from build123d import *

# Parameters (mm, degrees)
SKETCH1_W      = 5
SKETCH1_H      = 4
SKETCH2_R      = 3
EXTRUDE1_DEPTH = 12
EXTRUDE2_DEPTH = 3
CHAMFER1_SIZE  = 0.6135
FILLET1_R      = 0.2


with BuildPart() as part:
    # Sketch1 → Revolve1 (revolve)
    with BuildSketch(Plane.XZ.offset(-21.5)):
        with Locations((-13, -2.4)):
            Rectangle(SKETCH1_W, SKETCH1_H)
    revolve(axis=Axis((-15.5, 21.5, -0.4), (0, 0, -1)))

    # Sketch2 → Extrude1 (add)
    with BuildSketch(Plane(origin=(0, 0, -4.4), x_dir=(-1, 0, 0), z_dir=(0, 0, -1))):
        with Locations((15.5, 21.5)):
            Circle(SKETCH2_R)
    extrude(amount=EXTRUDE1_DEPTH)

    # Sketch3 → Extrude2 (cut)
    with BuildSketch(Plane.XY.offset(-0.4)):
        Polygon((-17.5, 22.654700538), (-17.5, 20.345299462), (-15.5, 19.190598923), (-13.5, 20.345299462), (-13.5, 22.654700538), (-15.5, 23.809401077), align=None)
    extrude(amount=-EXTRUDE2_DEPTH, mode=Mode.SUBTRACT)

    # Sketch4 → Cut-Revolve1 (revolve, cut)
    with BuildSketch(Plane.XZ.offset(-21.5)):
        Polygon((-13.5, -3.4), (-15.5, -3.4), (-15.5, -4.127940469), align=None)
    revolve(axis=Axis((-15.5, 21.5, -3.399975), (0, 0, -1)), mode=Mode.SUBTRACT)

    # Chamfer1
    chamfer1_edges = [part.edges().sort_by_distance(p)[0] for p in [
        (-12.5, 21.5, -16.4),
    ]]
    chamfer(chamfer1_edges, length=CHAMFER1_SIZE)

    # Fillet1
    fillet1_edges = [part.edges().sort_by_distance(p)[0] for p in [
        (-12.5, 21.5, -4.4),
    ]]
    fillet(fillet1_edges, radius=FILLET1_R)


solid = part.part
Geometry check sheet. Reference: the model listing, model coordinates, mm. A direction names the side the tool comes from. Round coordinates to 2 decimals unless told otherwise and drop trailing zeros. Order: outer loops, then holes, each group sorted by start corner. A loop starts at its lowest first (then second) coordinate and runs counter-clockwise, first axis right, second up. Notation, with made-up numbers: M 39,75.25 L 51,75.25 A21 ccw 51,107.25 Z; hole C 10.5,89 d3. An arc over 180 degrees is marked long. Write each question's results on one line, items separated by ' | '. Start each with the question number.
1. Cross-section at B-B on y = 18. Record the boundary of the cut face in (x, z).
2. Go/stop test with flat-tipped pins: P1, Ø0.7, axis at y = 22, z = -2.5, coming from the +X side; P2, Ø4, axis at y = 24, z = -6.5, coming from the +X side; P3, Ø6, axis at y = 19.5, z = -9.5, coming from the -X side. Record where each tip stops, or that it passes through.
3. Set-up check for faces 1 (the face through (-18, 21, -0.4)), 2 (the face through (-15, 25, -4.4)), 3 (the face through (-14.51, 19.76, -1.88)): record each of +Z, -Z, +X, -X, +Y, -Y from which the full face is reachable in a straight line by a thin tool's end or side.
4. Material ranges on L1, parallel to Z at x = -14.25, y = 17.5; L2, parallel to Y at x = -13.75, z = -2; L3, parallel to X at y = 17.5, z = -1.75, recorded low to high. Write a range as from..to.
5. Cross-section at A-A on z = -13.5. Record the boundary of the cut face in (x, y).
6. Draft check along X on faces 4 (the face through (-16.58, 26.38, -2.37)), 5 (the face through (-15.527, 21.622, -4.082)), 6 (the face through (-15, 22, -16.4)). Enter one of: pulls with the +X half, pulls with the -X half, needs draft (parallel to the pull), parting line crosses it, or undercut.
Resolved:
1) outline: M -19.07,-4.4 L -11.93,-4.4 L -11.93,-0.4 L -19.07,-0.4 Z
2) P1: x = -10.5 | P2: x = -12.54 | P3: x = -18.5
3) face 1: +Z, +X, -X, +Y, -Y | face 2: -Z | face 3: +Z
4) L1: -4.4..-0.4 | L2: 16.82..20.2, 22.8..26.18 | L3: -18.5..-12.5
5) outline: C -15.5,21.5 d6
6) face 4: parting line crosses it | face 5: undercut | face 6: needs draft
